Autodesk Inventor part; units mm, degrees
ref_plane "Work Plane1" through (29, 0, 0) normal (0, -1, 0) x (1, 0, 0)
ref_plane "YZ Plane" through (0, 0, 0) normal (1, 0, 0) x (0, 1, 0)
ref_plane "XZ Plane" through (0, 0, 0) normal (0, 1, 0) x (-1, 0, 0)
sketch "Sketch1" plane through (0, 0, 0) normal (0, 0, 1) x (1, 0, 0)
  line L0 (-0.9567, 0) -> (7.9375, 0)
  line L1 (7.9375, 0) -> (7.9375, 1.7526)
  line L2 (7.9375, 1.7526) -> (1.9847, 1.7526)
  line L3 (1.9847, 1.7526) -> (0.0001, 1.7526)
  line L4 (0.0001, 1.7526) -> (0, 1.7526)
  line L5 (0, 1.7526) -> (0, 2.8702)
  line L6 (0, 2.8702) -> (-3.5052, 2.8702)
  line L7 (-3.5052, 2.8702) -> (-3.5052, 1.5985)
  line L8 (-3.5052, 1.5985) -> (-1.8796, 1.5985)
  line L9 (-1.8796, 1.5985) -> (-0.9567, 0)
  line L10 (-5.7937, 0) -> (10.226, 0)
  line L11 (0, -0.574) -> (0, 3.4442)
  line L12 (1.9847, 1.7526) -> (0, 1.7526) construction
  dimension "d1" = 5.9528
  dimension "d2" = 1.9846
  dimension "d3" = 3.5052
  dimension "d4" = 1.6256
  dimension "d5" = 60
  dimension "d6" = 3.5052
  dimension "d7" = 3.5052
  dimension "d8" = 3.1969
  dimension "d9" = 5.7404
  dimension "d26" = 7.9375
revolve "Body" add sketch "Sketch1" angle 360 about axis through (-0.9567, 0, 0) along (1, 0, 0)
sketch "Sketch2" plane through (-3.5052, 0, 0) normal (-1, 0, 0) x (0, 0, 1)
  circle A0 centre (0, 0) radius 1.5985
  line L0 (0, -4.0183) -> (0, 4.0183)
  line L1 (-4.0183, 0) -> (4.0183, 0)
  line L2 (1.5985, 0) -> (0.7992, -1.3843)
  line L3 (0.7992, -1.3843) -> (-0.7992, -1.3843)
  line L4 (-0.7992, -1.3843) -> (-1.5985, 0)
  line L5 (-1.5985, 0) -> (-0.7992, 1.3843)
  line L6 (-0.7992, 1.3843) -> (0.7992, 1.3843)
  line L7 (0.7992, 1.3843) -> (1.5985, 0)
extrude "Slot" add sketch "Sketch2" against normal up to next contours L7 A0 | A0 L2 | L6 L0 A0 | A0 L0 L3 | L0 L6 A0 | A0 L3 L0 | L4 A0 | A0 L5
fillet "Fillet1" radius 0.3302 1 edges at (-3.5052, -2.8702, 0)
thread "Thread"
chamfer "Chamfer1" distance 0.4724 distance2 0.4724 1 edges at (7.9375, -1.7526, 0) measured on face at (7.9375, -0.5672, -0.1398)
ref_plane "Work Plane1" through (29, 0, 0) normal (0, -1, 0) x (1, 0, 0)
fillet "Fillet2" radius 0.127 1 edges at (0.0001, -1.7526, 0)
equation "\"d1\" = GEL"
equation "\"d3\" = KOH"
equation "\"d4\" = INTI"
equation "\"d6\" = GD"
equation "\"d7\" = BDM"
equation "\"d8\" = 1.1547 * SW"
equation "\"d9\" = KOD"
equation "\"d26\" = NLG"
equation "\"d30\" = R"
equation "\"d17\" = RR"
equation "\"d13\" = GEL"
equation "\"d15\" = -0.5 * SPD + 0.5 * GD"
equation "\"d16\" = GUL"
equation "\"GD\" = 3.5052"
equation "\"NLG\" = 7.9375"
equation "\"GEL\" = 5.9528"
equation "\"KOD\" = 5.7404"
equation "\"KOH\" = 3.5052"
equation "\"INTI\" = 1.6256"
equation "\"GAL\" = 1.9845"
equation "\"GUL\" = 0.47244"
equation "\"BDM\" = 3.5052"
equation "\"SW\" = 2.7686"
equation "\"RR\" = 0.3302"
equation "\"SPD\" = 2.56032"
equation "\"R\" = 0.127"
equation "\"PHH\" = 0.127"
equation "\"GD1\" = SPD"
equation "\"THREADDIA\" = 3.5052"
equation "\"FAWI\" = 45deg"
equation "\"KOH1\" = 3.1496"
equation "\"NND\" = 3.5052"
equation "\"TOA\" = 30deg"
equation "\"E0\" = 1.155 * SW"
properties part number "ANSI B18.3 - No. 6 - 32 UNC - 5/16 HS HCS" material "Steel, Mild"
Design review of the part built by this model. Coordinates are the model's own, in mm. A direction names the side the tool comes from. Give positions to 0.01 mm unless a question says otherwise; leave off trailing zeros. Order: outer loops, then holes, each group sorted by start corner. A loop starts at its lowest first (then second) coordinate and runs counter-clockwise, first axis right, second up. Notation, with made-up numbers: (48, 48) - (104, 48) arc R21 ccw to (104, 73) - close; hole circle Ø11 at (10, 24). An arc over 180 degrees is marked (long way). Use a Markdown table: item, result. Add a question column.
(1) Clearance check with a flat-ended pin moving along its axis: P1, Ø1.5, axis at x = 2, z = -0.5, coming from the -Y side. State where the tip first meets the part, or that it passes through.
(2) Add section B-B on x = 5. Give the boundary of the cut face in (y, z), then the cut area to 3 significant figures.
(3) Add section A-A on x = -2. Give the boundary of the cut face in (y, z).
(4) Wall thickness on probe 1 along Z at (x, y) = (0.75, 1.2); probe 2 along X at (y, z) = (-2.15, 0.25); probe 3 along Y at (x, z) = (-2, -0.6): over which ranges is each line inside the solid? List them lowest first. Write a range as [from, to].
(5) Mouldability with a two-part tool opening along Y and no side actions: class faces 4 (the face through (-3, 1.384, 0)), 5 (the face through (0, 1, 2)), 6 (the face through (-1.014, 0.095, -0.03)), 7 (the face through (-1.61, -2.278, 1.746)) as +Y half, -Y half, draft (parallel to the pull), parting line (faces both ways), or undercut.
(6) Machinability: for faces 1 (the face through (3.745, -1.292, -1.184)), 2 (the face through (-3.505, -2, 0)), 3 (the face through (-2.643, 0.702, 1.193)), which of the approach directions +Z, -Z, +X, -X, +Y, -Y give a long, thin tool a straight path to every point of the face, cutting with its end or side? Answer none if there is none.
Report:
| question | item | result |
|---|---|---|
| 1 | P1 | stops at y = -1.75 |
| 2 | outline | circle Ø3.51 at (0, 0) |
| 2 | area | 9.65 mm² |
| 3 | outline | circle Ø5.74 at (0, 0); hole (-1.38, -0.8) - (0, -1.6) - (1.38, -0.8) - (1.38, 0.8) - (0, 1.6) - (-1.38, 0.8) - close |
| 4 | probe 1 | z = [-1.28, 1.28] |
| 4 | probe 2 | x = [-3.51, 0] |
| 4 | probe 3 | y = [-2.81, -1.38], [1.38, 2.81] |
| 5 | face 4 | undercut |
| 5 | face 5 | draft |
| 5 | face 6 | undercut |
| 5 | face 7 | parting line |
| 6 | face 1 | +X |
| 6 | face 2 | +Z, -Z, -X, +Y, -Y |
| 6 | face 3 | -X |
